The figure shows three views and two pictorial views of one solid part (mm, origin at its lowest corner). Answer the questions. Coordinates: 2 decimals unless noted, no trailing zeros. Loops run counter-clockwise (first coordinate to the right, second up) from the corner with the lowest first, then second, coordinate; pieces in that order, holes last.
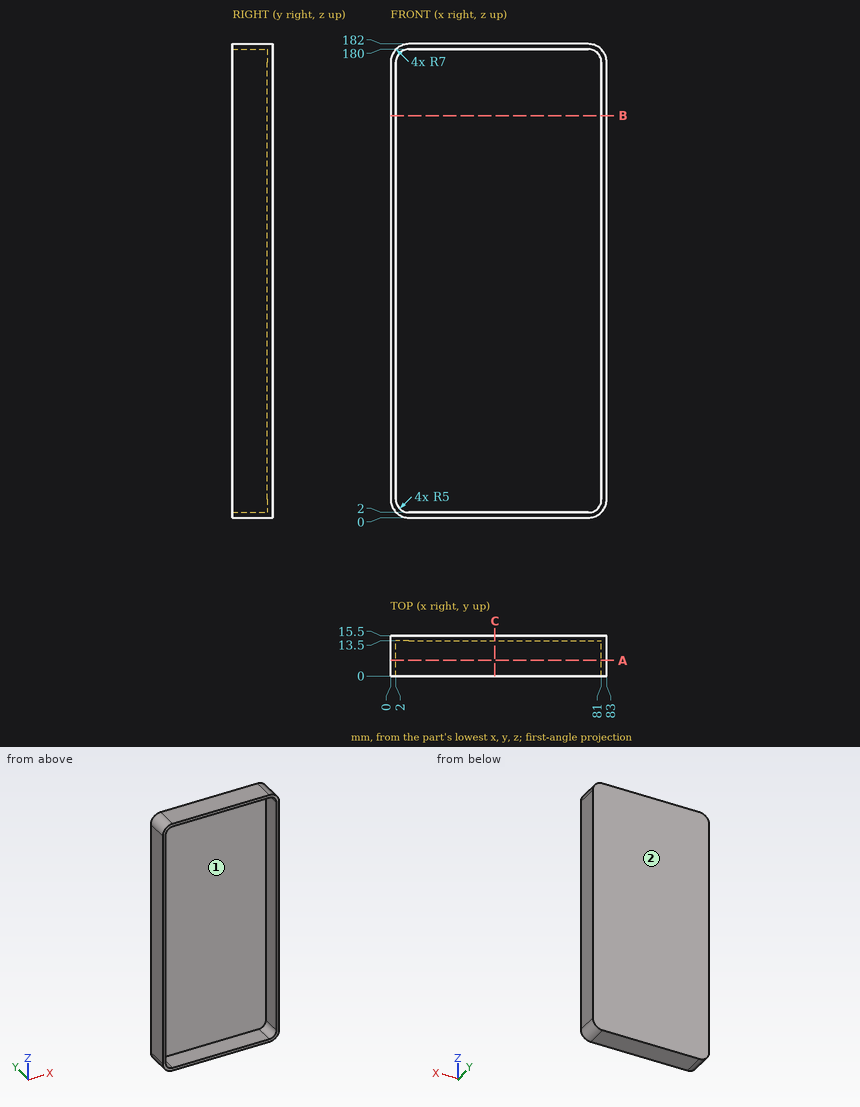
Q1. A cutting plane is placed at C-C (x = 40). Give the vertices of the cut face in (y, z), then the cut area to 3 significant figures.
Findings below:
outline: (0, 0) - (15.5, 0) - (15.5, 182) - (0, 182) - (0, 180) - (13.5, 180) - (13.5, 2) - (0, 2) - close
area: 418 mm2
Q2. Straight lines are drawn through the part: probe 1 along X at (y, z) = (5, 156); probe 2 along Z at (x, y) = (14, 13); probe 3 along Y at (x, z) = (58.5, 124.5). For each, find the intervals that lie inside material, in ascending order.
Findings below:
probe 1: x = 0 to 2, 81 to 83
probe 2: z = 0 to 2, 180 to 182
probe 3: y = 13.5 to 15.5
Q3. A flat-ended cylindrical pin translates along its axis: pin 1 Ø23.5 at (x, z) = (56.5, 125) entering from -Y. Find the tip coordinate at first contact, or state that the pin passes through.
Findings below:
pin 1: stops at y = 13.5
Q4. Determine the mould class of the marked faces 1 and 2 for opening direction X: +X half, -X half, draft (parallel to the pull), parting line (faces both ways), or undercut.
Findings below:
face 1: undercut
face 2: draft
Q5. A cutting plane is placed at A-A (y = 6). Give the vertices of the cut face in (x, z), then the cut area to 3 significant figures.
Findings below:
outline: (0, 7) arc R7 ccw to (7, 0) - (76, 0) arc R7 ccw to (83, 7) - (83, 175) arc R7 ccw to (76, 182) - (7, 182) arc R7 ccw to (0, 175) - close; hole (2, 7) arc R5 ccw to (7, 2) - (76, 2) arc R5 ccw to (81, 7) - (81, 175) arc R5 ccw to (76, 180) - (7, 180) arc R5 ccw to (2, 175) - close
area: 1,020 mm2
Q6. A cutting plane is placed at B-B (z = 154.5). Give the vertices of the cut face in (x, y).
Findings below:
outline: (0, 0) - (2, 0) - (2, 13.5) - (81, 13.5) - (81, 0) - (83, 0) - (83, 15.5) - (0, 15.5) - close
